For this review, take the finished solid that the model builds, in its own axes (mm). A direction names the side the tool comes from. Coordinates: 2 decimals unless noted, no trailing zeros. Loops run counter-clockwise (first coordinate to the right, second up) from the corner with the lowest first, then second, coordinate; pieces in that order, holes last.
1. To check wall thickness, follow probe 1 along Y at (x, z) = (-22.5, 0.2); probe 2 along X at (y, z) = (-13.5, 1.35); probe 3 along X at (y, z) = (-12.5, 0.6). State the ranges of each line that lie inside material, in increasing order.
2. Machinability: for faces 1 (the face through (52.073, -25.67, 0.986)), 2 (the face through (-45.08, -10.98, 0.99)), which of the approach directions +Z, -Z, +X, -X, +Y, -Y give a long, thin tool a straight path to every point of the face, cutting with its end or side? Answer none if there is none.
3. Take a section at D-D, the plane x = 53.5. State the section outline as (y, z) points, then the cut area to 3 significant figures.
4. Take a section at C-C, the plane x = -66. State the section outline as (y, z) points.
5. Clearance check with a flat-ended pin moving along its axis: P1, Ø3, axis at x = 43, y = -9.5, coming from the -Z side. State where the tip first meets the part, or that it passes through.
6. Take a section at B-B, the plane z = 0.9. Count the separate pieces of the cut face and the enclosed holes in it, then the cut area to 3 significant figures.
7. Mouldability with a two-part tool opening along X and no side actions: class faces 3 (the face through (73.684, 1, 0.986)), 4 (the face through (-1, -13, 0)), 5 (the face through (-5, -11, 1)), 6 (the face through (-52.229, -25.515, 0.986)) as pulls with the +X half, pulls with the -X half, needs draft (parallel to the pull), parting line crosses it, or undercut.
8. Take a section at A-A, the plane x = 13.5. State the section outline as (y, z) points.
```python
from build123d import *

# Parameters (mm, degrees)
SKETCH1_W           = 80
SKETCH1_H           = 3
BOSS_EXTRUDE1_DEPTH = 2


with BuildPart() as part:
    # Sketch1 → Boss-Extrude1 (new body)
    # profile 1 of 2: a face of its own
    with BuildSketch(Plane.XY):
        with BuildLine():
            Line((-75.109333092, -2.496355564), (-75.109333092, -2.503644436))
            Line((-75.109333092, -2.503644436), (-55.0801776, -2.478133382))
            Line((-55.0801776, -2.478133382), (-55.0801776, -18.521866618))
            ThreePointArc((-55.0801776, -18.521866618), (-52.151245412, -25.59293443), (-45.0801776, -28.521866618))
            Line((-45.0801776, -28.521866618), (45.0801776, -28.521866618))
            ThreePointArc((45.0801776, -28.521866618), (52.151245412, -25.59293443), (55.0801776, -18.521866618))
            Line((55.0801776, -18.521866618), (55.0801776, -2.478133382))
            Line((55.0801776, -2.478133382), (75.109333092, -2.503644436))
            Line((75.109333092, -2.503644436), (75.109333092, -2.496355564))
            ThreePointArc((75.109333092, -2.496355564), (73.644866997, 1.039178342), (70.109333092, 2.503644436))
            Line((70.109333092, 2.503644436), (-70.109333092, 2.503644436))
            Line((-70.109333092, 2.503644436), (-75.109333092, 2.503644436))
            Line((-75.109333092, 2.503644436), (-75.109333092, -2.496355564))
        make_face()
        with Locations((0, -22.521866618)):
            Rectangle(SKETCH1_W, SKETCH1_H, mode=Mode.SUBTRACT)
        with BuildLine():
            ThreePointArc((-40.0801776, -15.868057699), (-45.0801776, -10.868057699), (-40.0801776, -5.868057699))
            Line((-40.0801776, -5.868057699), (-10, -5.868057699))
            ThreePointArc((-10, -5.868057699), (-5, -10.868057699), (-10, -15.868057699))
            Line((-10, -15.868057699), (-40.0801776, -15.868057699))
        make_face(mode=Mode.SUBTRACT)
        with BuildLine():
            ThreePointArc((10, -15.868057699), (5, -10.868057699), (10, -5.868057699))
            Line((10, -5.868057699), (40.0801776, -5.868057699))
            ThreePointArc((40.0801776, -5.868057699), (45.0801776, -10.868057699), (40.0801776, -15.868057699))
            Line((40.0801776, -15.868057699), (10, -15.868057699))
        make_face(mode=Mode.SUBTRACT)
    # profile 2 of 2: a face of its own
    with BuildSketch(Plane.XY):
        with BuildLine():
            Line((-75.109333092, -2.496355564), (-75.109333092, -2.503644436))
            Line((-75.109333092, -2.503644436), (-55.0801776, -2.478133382))
            Line((-55.0801776, -2.478133382), (-55.0801776, -18.521866618))
            ThreePointArc((-55.0801776, -18.521866618), (-52.151245412, -25.59293443), (-45.0801776, -28.521866618))
            Line((-45.0801776, -28.521866618), (45.0801776, -28.521866618))
            ThreePointArc((45.0801776, -28.521866618), (52.151245412, -25.59293443), (55.0801776, -18.521866618))
            Line((55.0801776, -18.521866618), (55.0801776, -2.478133382))
            Line((55.0801776, -2.478133382), (75.109333092, -2.503644436))
            Line((75.109333092, -2.503644436), (75.109333092, -2.496355564))
            ThreePointArc((75.109333092, -2.496355564), (73.644866997, 1.039178342), (70.109333092, 2.503644436))
            Line((70.109333092, 2.503644436), (-70.109333092, 2.503644436))
            Line((-70.109333092, 2.503644436), (-75.109333092, 2.503644436))
            Line((-75.109333092, 2.503644436), (-75.109333092, -2.496355564))
        make_face()
        with Locations((0, -22.521866618)):
            Rectangle(SKETCH1_W, SKETCH1_H, mode=Mode.SUBTRACT)
        with BuildLine():
            ThreePointArc((-40.0801776, -15.868057699), (-45.0801776, -10.868057699), (-40.0801776, -5.868057699))
            Line((-40.0801776, -5.868057699), (-10, -5.868057699))
            ThreePointArc((-10, -5.868057699), (-5, -10.868057699), (-10, -15.868057699))
            Line((-10, -15.868057699), (-40.0801776, -15.868057699))
        make_face(mode=Mode.SUBTRACT)
        with BuildLine():
            ThreePointArc((10, -15.868057699), (5, -10.868057699), (10, -5.868057699))
            Line((10, -5.868057699), (40.0801776, -5.868057699))
            ThreePointArc((40.0801776, -5.868057699), (45.0801776, -10.868057699), (40.0801776, -15.868057699))
            Line((40.0801776, -15.868057699), (10, -15.868057699))
        make_face(mode=Mode.SUBTRACT)
    extrude(amount=BOSS_EXTRUDE1_DEPTH)


solid = part.part
```
Results list:
1. probe 1: y = -28.52 to -24.02, -21.02 to -15.87, -5.87 to 2.5
1. probe 2: x = -55.08 to -44.33, -5.75 to 5.75, 44.33 to 55.08
1. probe 3: x = -55.08 to -44.81, -5.27 to 5.27, 44.81 to 55.08
2. face 1: +Z, -Z, +X, -Y
2. face 2: +Z, -Z
3. outline: (-23.92, 0) - (2.5, 0) - (2.5, 2) - (-23.92, 2) - close
3. area: 52.8 mm2
4. outline: (-2.49, 0) - (2.5, 0) - (2.5, 2) - (-2.49, 2) - close
5. P1: passes through
6. separate pieces: 1
6. enclosed holes: 3
6. area: 2,570 mm2
7. face 3: pulls with the +X half
7. face 4: needs draft
7. face 5: undercut
7. face 6: pulls with the -X half
8. outline: (-28.52, 0) - (-24.02, 0) - (-24.02, 2) - (-28.52, 2) - close; (-21.02, 0) - (-15.87, 0) - (-15.87, 2) - (-21.02, 2) - close; (-5.87, 0) - (2.5, 0) - (2.5, 2) - (-5.87, 2) - close
